Autodesk Fusion 360 part; units mm, degrees
sketch "Sketch1" plane through (0, 0, 0) normal (1, 0, 0) x (0, 0, -1)
  line L0 (0, 0) -> (0, 45)
  line L1 (0, 0) -> (0, -45)
  line L2 (0, 45) -> (37.5, 45)
  line L3 (0, 45) -> (-37.5, 45)
  line L4 (0, -45) -> (37.5, -45)
  line L5 (0, -45) -> (-37.5, -45)
  arc A0 (-37.5, 45) -> (-37.5, -45) centre (79.119, 0) ccw
  arc A1 (37.5, -45) -> (37.5, 45) centre (-79.119, 0) ccw
  dimension "d1" = 45
  dimension "d2" = 45
  dimension "d3" = 37.5
  dimension "d4" = 37.5
  dimension "d5" = 37.5
  dimension "d6" = 37.5
  dimension "d8" = 125
extrude "Extrude1" add sketch "Sketch1" along normal blind 100
extrude "Extrude2" add 1 faces at (100, -15.2642, -14.2806) along direction (1, 0, 0) blind 35 draft -15
sketch "Sketch2" plane through (135, 0, 0) normal (1, 0, 0) x (0, 0, -1)
  line L0 (-30.8786, -35.6218) -> (30.8786, -35.6218)
  arc A0 (30.8786, -35.6218) -> (30.8786, 35.6218) centre (-79.119, 0) ccw
  line L1 (30.8786, 35.6218) -> (-30.8786, 35.6218)
  arc A1 (-30.8786, 35.6218) -> (-30.8786, -35.6218) centre (79.119, 0) ccw
  circle A2 centre (0, 0) radius 34.5
  dimension "d13" = 69
extrude "Extrude3" add sketch "Sketch2" along normal blind 10 contours A2
sketch "Sketch3" plane through (145, 0, 0) normal (1, 0, 0) x (0, 0, -1)
  circle A0 centre (0, 0) radius 34.5
  circle A1 centre (0, 0) radius 31
  dimension "d16" = 62
extrude "Extrude4" add sketch "Sketch3" along normal blind 30 contours A1
sketch "Sketch4" plane through (175, 0, 0) normal (1, 0, 0) x (0, 0, -1)
  circle A0 centre (0, 0) radius 31
  line L0 (0, 0) -> (27, 0)
  circle A1 centre (27, 0) radius 2.5
  circle A2 centre (27, 0) radius 1.5
  dimension "d19" = 27
  dimension "d20" = 5
  dimension "d21" = -1
extrude "Extrude5" add sketch "Sketch4" along normal blind 1 contours A1
pattern_circular "C-Pattern1" count 12 over 360 about axis through (175, 0, 0) along (1, 0, 0) of "Extrude5"
sketch "Sketch5" plane through (175, 0, 0) normal (1, 0, 0) x (0, 0, -1)
  circle A0 centre (27, 0) radius 2.5
  circle A1 centre (0, 0) radius 31
  circle A2 centre (23.3827, 13.5) radius 2.5
  circle A3 centre (13.5, 23.3827) radius 2.5
  circle A4 centre (0, 27) radius 2.5
  circle A5 centre (-13.5, 23.3827) radius 2.5
  circle A6 centre (-23.3827, 13.5) radius 2.5
  circle A7 centre (-27, 0) radius 2.5
  circle A8 centre (-23.3827, -13.5) radius 2.5
  circle A9 centre (-13.5, -23.3827) radius 2.5
  circle A10 centre (0, -27) radius 2.5
  circle A11 centre (13.5, -23.3827) radius 2.5
  circle A12 centre (23.3827, -13.5) radius 2.5
  line L0 (0, 0) -> (16, 0)
  line L1 (16, 0) -> (16, 17)
  line L2 (16, 0) -> (16, -17)
  line L3 (0, 0) -> (0, -8.0593)
  line L4 (-16, 0) -> (-16, 17)
  line L5 (-16, 0) -> (-16, -17)
  arc A13 (16, 17) -> (-16, 17) centre (0, 1.9003) ccw
  arc A14 (-16, -17) -> (16, -17) centre (0, -1.9003) ccw
  dimension "d26" = 16
  dimension "d27" = 17
  dimension "d28" = 17
  dimension "d29" = 22
extrude "Extrude6" add sketch "Sketch5" along normal blind 100 contours L1 L2 L4 L5 A13 A14
sketch "Sketch6" plane through (275, 0, 0) normal (1, 0, 0) x (0, 0, -1)
  line L0 (-16, 17) -> (-16, -17)
  arc A0 (-16, -17) -> (16, -17) centre (0, -1.9003) ccw
  line L1 (16, -17) -> (16, 17)
  arc A1 (16, 17) -> (-16, 17) centre (0, 1.9003) ccw
  circle A2 centre (0, 0) radius 31
  circle A3 centre (0, 0) radius 30
  dimension "d32" = 62
  dimension "d35" = -1
extrude "Extrude7" add sketch "Sketch6" along normal blind 10 contours L0 A0 L1 A1 | A2 | A3
sketch "Sketch7" plane through (285, 0, 0) normal (1, 0, 0) x (0, 0, -1)
  circle A0 centre (0, 0) radius 31
  circle A1 centre (0, 0) radius 30
  dimension "d36" = -1
extrude "Extrude8" add sketch "Sketch7" along normal blind 1 contours A1
sketch "Sketch8" plane through (286, 0, 0) normal (1, 0, 0) x (0, 0, -1)
  circle A0 centre (0, 0) radius 30
  circle A1 centre (0, 0) radius 31
  dimension "d39" = 62
extrude "Extrude9" add sketch "Sketch8" along normal blind 10 contours A0 | A1
ref_plane "WorkPlane1" through (0, 45, 37.5) normal (0, 0, 1) x (1, 0, 0)
sketch "Sketch9" plane through (0, 0, 37.5) normal (0, 0, 1) x (1, 0, 0)
  circle A0 centre (50, -45) radius 42.5
  dimension "d43" = 85
extrude "Extrude10" add sketch "Sketch9" along normal mid plane 21
sketch "Sketch10" plane through (0, 0, 27) normal (0, 0, -1) x (-1, 0, 0)
  line L0 (-7.5, -45) -> (-92.5, -45)
  arc A0 (-92.5, -45) -> (-7.5, -45) centre (-50, -45) ccw
  line L1 (-50, -45) -> (-50, -75)
  line L2 (-70, -45) -> (-70, -74.9351)
  line L3 (-30, -45) -> (-30, -74.738)
  arc A1 (-70, -74.9351) -> (-30, -74.738) centre (-50.1102, -52.4763) ccw
  dimension "d46" = 30
  dimension "d47" = 20
  dimension "d48" = -20
  dimension "d49" = 30
extrude "Extrude11" add sketch "Sketch10" along normal blind 35 contours L0 L2 L3 A1
equation "d44 = ( 21 / 2 ) * 1 mm"
Read the model definition and answer for the solid it produces. Units are mm, in the model's axes. A direction names the side the tool comes from. Give positions to 0.01 mm unless a question says otherwise; leave off trailing zeros. Write each loop counter-clockwise with the first axis right and the second up, starting at its lowest first coordinate (ties: lowest second). Pieces come first, ordered by that corner, then holes. Notation, with made-up numbers: (-35.75, 86) - (3.25, 86) arc R16 ccw to (3.25, 115) - close; hole circle Ø2 at (52, 65.5). An arc over 180 degrees is marked (long way). Return JSON: item names as keys, results as strings.
Q1. For a pull along X with two mould halves and no side action, classify faces 1 (the face through (275, 0, -20)), 2 (the face through (279.93, -30.736, 4.036)), 3 (the face through (117.255, -0.621, 41.256)), 4 (the face through (224, 0, -16)) as released by +X, released by -X, zero draft, split by the parting line, or undercut.
Reply:
{"face 1": "undercut", "face 2": "zero draft", "face 3": "released by +X", "face 4": "undercut"}
Q2. Consider line 1 along Z through (x, y) = (175.75, 13.5); line 2 along X through (y, z) = (2, 30.5); line 3 along X through (y, z) = (-16, -24). Determine where each line is inside the solid, lowest interval first. Write a range as [from, to].
Reply:
{"line 1": "[-25.88, -24.88], [-21.88, -20.88], [-16, 16], [20.88, 21.88], [24.88, 25.88]", "line 2": "[0, 175], [275, 285], [286, 296]", "line 3": "[0, 175], [275, 296]"}
Q3. A cutting plane is placed at C-C, the plane y = -50. Determine the outline of the cut face in (x, z).
Reply:
{"outline": "(7.8, 27) - (30, 27) - (30, -8) - (70, -8) - (70, 27) - (92.2, 27) - (92.2, 48) - (7.8, 48) - close"}
Q4. A cutting plane is placed at A-A, the plane y = -64.5. Determine the outline of the cut face in (x, z), and give its area (3 significant figures).
Reply:
{"outline": "(12.24, 27) - (30, 27) - (30, -8) - (70, -8) - (70, 27) - (87.76, 27) - (87.76, 48) - (12.24, 48) - close", "area": "2,990 mm²"}
Q5. A cutting plane is placed at D-D, the plane x = 33. Determine the outline of the cut face in (y, z), and give its area (3 significant figures).
Reply:
{"outline": "(-83.95, 27) - (-77.12, 27) - (-77.12, -8) - (-45, -8) - (-45, -37.5) arc R125 ccw to (45, -37.5) - (45, 37.5) arc R125 ccw to (-6.05, 45.73) - (-6.05, 48) - (-83.95, 48) - close", "area": "9,910 mm²"}
Q6. A cutting plane is placed at B-B, the plane x = 140. Determine the outline of the cut face in (y, z).
Reply:
{"outline": "circle Ø69 at (0, 0)"}
Q7. For faces 5 (the face through (50, -63, -8)), 6 (the face through (285, 28, 12)), 7 (the face through (139.93, -10.363, -32.907)), 8 (the face through (70, -60, 10)), 9 (the face through (43.5, -81.9, 27)), determine the directions among +Z, -Z, +X, -X, +Y, -Y from which every point of the face is accessible in a straight line to the end or side of a thin tool.
Reply:
{"face 5": "-Z, +X, -X, -Y", "face 6": "none", "face 7": "+X", "face 8": "-Z, +X, -Y", "face 9": "-Z, -Y"}
Q8. Given P1, Ø24, axis at y = -63.5, z = 12.5, coming from the +X side; P2, Ø1.5, axis at x = 66, y = 9.5, coming from the -Z side; P3, Ø1, axis at y = -59.5, z = 21.5, coming from the -X side, each flat-ended and moving along its own axis, determine where each tip first touches the part or whether it passes through.
Reply:
{"P1": "x = 70", "P2": "z = -45.57", "P3": "x = 30"}
